Build history of the part. All positions in model axes, mm. Face numbers are marked on the shaded views. Give positions to 0.01 mm unless a question says otherwise; leave off trailing zeros. Loops run counter-clockwise (first coordinate to the right, second up) from the corner with the lowest first, then second, coordinate; pieces in that order, holes last. Notation, with made-up numbers: (-8, 47) - (10, 47) arc R5 ccw to (10, 51) - close; hole circle Ø4 at (3, -10.5). An arc over 180 degrees is marked (long way). Return JSON: item names as keys, results as strings. Group by question number.
1) Drill centre lines: probe 1 along Y at (x, z) = (0, 11.75); probe 2 along Y at (x, z) = (-2.25, 12.75); probe 3 along X at (y, z) = (-7.25, 14.75). Where is each one in solid material? Low to high. Write a range as from..to.
2) Drop flat-ended pins along their axis: pin 1 (3 mm diameter, centred on y = -3, z = 14.5, fed in from -X); pin 2 (7 mm diameter, centred on x = 0, y = 0, fed in from +Z). Give the stop position or say it passes through.
3) Slice it at C-C (z = 10.75). List the corners of the cut face in (x, y).
4) Mould opens along X. For the marked faces 1, 2 and 3 say: released by +X, released by -X, zero draft, split by the parting line, or undercut.
```python
from build123d import *

# Parameters (mm, degrees)
SKETCH002_R   = 11
SKETCH002_R_2 = 4
PAD002_DEPTH  = 3.5


with BuildPart() as part:
    # Sketch002 → Pad002 (new body, symmetric)
    with BuildSketch(Plane.XY):
        Circle(SKETCH002_R)
        Circle(SKETCH002_R_2, mode=Mode.SUBTRACT)
    extrude(amount=PAD002_DEPTH, both=True)

    # Sketch003 → Groove (revolve, cut)
    with BuildSketch(Plane.YZ):
        Polygon((3.265378, -9.726486), (6, -3.124525), (6.615998, -4.611675), (9.384002, -4.611675), (10, -3.124525), (10.963347, -5.45025), (14.375534, -9.430194), (8.874444, -10.64642), align=None)
    groove = revolve(axis=Axis((0, 0, 0), (0, 0, 1)), mode=Mode.SUBTRACT)

    # Mirrored: Groove across XY
    add(groove.mirror(Plane.XY), mode=Mode.SUBTRACT)


with BuildPart() as part_1:
    # Body001 placement: moved
    add(part.part.moved(Location((0, 0, 12.75))))


solid = part_1.part
```
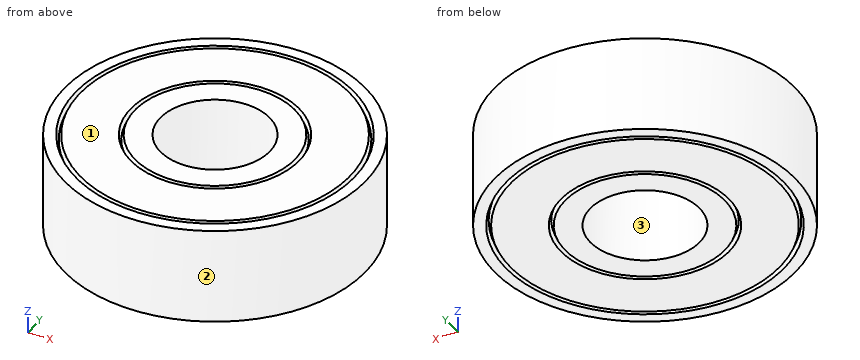
Results:
{
 "1": {"probe 1": "-11..-4, 4..11", "probe 2": "-10.77..-3.31, 3.31..10.77", "probe 3": "-8.27..8.27"},
 "2": {"pin 1": "x = -10.9", "pin 2": "through"},
 "3": {"outline": "circle Ø22 at (0, 0); hole circle Ø8 at (0, 0)"},
 "4": {"face 1": "zero draft", "face 2": "split by the parting line", "face 3": "undercut"}
}
